```python
from build123d import *

# Parameters (mm, degrees)
EXTRUDE_1_DEPTH = 5
SKETCH_3_W      = 9.6
SKETCH_3_H      = 10
SKETCH_3_R      = 2.5
EXTRUDE_2_DEPTH = 5
FILLET_1_R      = 1


with BuildPart() as part:
    # 草图1 → 凸台-拉伸1 (new, symmetric)
    with BuildSketch(Plane.XY):
        with BuildLine():
            Line((12.447157347, 0.266033793), (14.4, 0.266033793))
            Line((14.4, 0.266033793), (14.4, 17.45))
            Line((14.4, 17.45), (-14.4, 17.45))
            Line((-14.4, 17.45), (-14.4, 0.266033793))
            Line((-14.4, 0.266033793), (-12.447157347, 0.266033793))
            ThreePointArc((-12.447157347, 0.266033793), (0, 12.45), (12.447157347, 0.266033793))
        make_face()
    extrude(amount=EXTRUDE_1_DEPTH, both=True)

    # 草图3 → 凸台-拉伸2 (add)
    # profile 1 of 2: a face of its own
    with BuildSketch(Plane.XZ.offset(-0.266033793)):
        with Locations((19.2, 0)):
            Rectangle(SKETCH_3_W, SKETCH_3_H)
        with Locations(Location((20, 0, 0), (0, 0, 90))):
            Circle(SKETCH_3_R, mode=Mode.SUBTRACT)
    # profile 2 of 2: a face of its own
    with BuildSketch(Plane.XZ.offset(-0.266033793)):
        with Locations((-19.2, 0)):
            Rectangle(SKETCH_3_W, SKETCH_3_H)
        with Locations(Location((-20, 0, 0), (0, 0, 270))):
            Circle(SKETCH_3_R, mode=Mode.SUBTRACT)
    extrude(amount=-EXTRUDE_2_DEPTH)

    # 圆角1
    fillet_1_edges = [part.edges().sort_by_distance(p)[0] for p in [
        (14.4, 5.266033793, 0),
        (-14.4, 5.266033793, 0),
    ]]
    fillet(fillet_1_edges, radius=FILLET_1_R)


solid = part.part
```
Design review of the part built by this model. Coordinates are the model's own, in mm. A direction names the side the tool comes from. Coordinates: 2 decimals unless noted, no trailing zeros. Loops run counter-clockwise (first coordinate to the right, second up) from the corner with the lowest first, then second, coordinate; pieces in that order, holes last.
Q1. To check wall thickness, follow line 1 (X direction, y = 2.2, z = 0); line 2 (X direction, y = 3.75, z = -1.5); line 3 (X direction, y = 16, z = 4). State the ranges of each line that lie inside material, in increasing order.
Reported:
line 1: x = -24 to -22.5, -17.5 to -12.25, 12.25 to 17.5, 22.5 to 24
line 2: x = -24 to -22, -18 to -11.87, 11.87 to 18, 22 to 24
line 3: x = -14.4 to 14.4
Q2. We need section B-B on y = 4.75. State the section outline as (x, z) points, and give its area (3 significant figures).
Reported:
outline: (-24, -5) - (-11.51, -5) - (-11.51, 5) - (-24, 5) - close; (11.51, -5) - (24, -5) - (24, 5) - (11.51, 5) - close; hole circle Ø5 at (-20, 0); hole circle Ø5 at (20, 0)
area: 211 mm2
Q3. Tool access review of faces 1 (the face through (17, 0.266, 0)), 2 (the face through (-14.4, 12, 0)), 3 (the face through (17, 5.266, 0)): name each direction out of +Z, -Z, +X, -X, +Y, -Y from which nothing blocks a thin tool from reaching the whole face with its end or side.
Reported:
face 1: +Z, -Z, +X, -X, -Y
face 2: +Z, -Z, -X, +Y
face 3: +Z, -Z, +X, +Y
Q4. The part is to be moulded in two halves that separate along X. For faces 4 (the face through (-14.685, 5.567, 0.07)), 5 (the face through (24, 3, 0)), 6 (the face through (17.52, 2.73, -0.33)), say which applies: +X half, -X half, draft (parallel to the pull), parting line (faces both ways), or undercut.
Reported:
face 4: -X half
face 5: +X half
face 6: undercut
Q5. For pin 1 (1 mm diameter, centred on x = -9, z = 2, fed in from -Y); pin 2 (5 mm diameter, centred on y = 13.5, z = 0, fed in from +X); pin 3 (3 mm diameter, centred on y = 9.5, z = -0.5, fed in from -X), all flat-tipped, find the tip position at first contact; note any pin that passes through.
Reported:
pin 1: stops at y = 8.05
pin 2: stops at x = 14.4
pin 3: stops at x = -14.4
Q6. We need section A-A on x = 20. State the section outline as (y, z) points.
Reported:
outline: (0.27, -5) - (5.27, -5) - (5.27, -2.5) - (0.27, -2.5) - close; (0.27, 2.5) - (5.27, 2.5) - (5.27, 5) - (0.27, 5) - close
